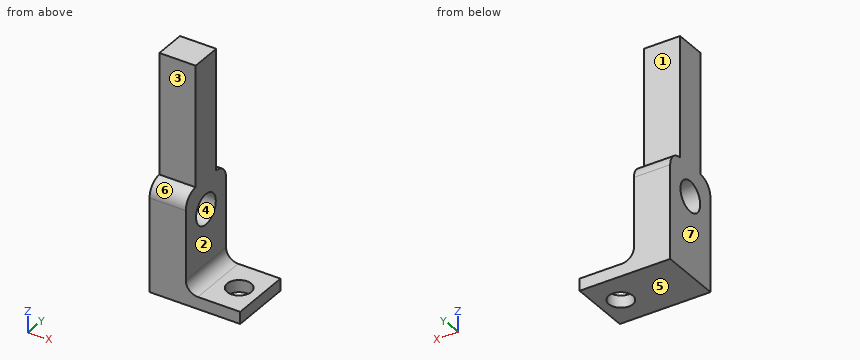
Autodesk Fusion 360 part; units mm, degrees
sketch "Sketch1" plane through (0, 0, 0) normal (0, 0, 1) x (1, 0, 0)
  line L0 (0, 0) -> (32, 0)
  line L1 (32, 0) -> (32, 10.2)
  line L2 (32, 10.2) -> (0, 10.2)
  line L3 (0, 10.2) -> (0, 0)
  dimension "d1" = 32
  dimension "d2" = 10.2
extrude "Extrude1" add sketch "Sketch1" along normal blind 2
sketch "Sketch2" plane through (0, 0, 2) normal (0, 0, 1) x (-1, 0, 0)
  line L0 (0, -10.2) -> (0, 0)
  line L1 (0, 0) -> (-32, 0)
  line L2 (-32, 0) -> (-32, -10.2)
  line L3 (-32, -10.2) -> (0, -10.2)
  line L4 (-7, -10.2) -> (-25, -10.2)
  line L5 (-25, -10.2) -> (-25, 0)
  line L6 (-25, 0) -> (-7, 0)
  line L7 (-7, 0) -> (-7, -10.2)
  circle A0 centre (-3.5, -5.1) radius 2
  circle A1 centre (-28.5, -5.1) radius 2
  dimension "d5" = 7
  dimension "d6" = 7
  dimension "d7" = 5.1
  dimension "d8" = 3.5
  dimension "d9" = 4
  dimension "d10" = 3.5
  dimension "d11" = 5.1
  dimension "d12" = 4
extrude "Extrude2" cut sketch "Sketch2" against normal blind 2.1 contours A0 | A1
extrude "Extrude3" add sketch "Sketch2" along normal blind 16 contours L1 L3 L4 L5 L6 L7
sketch "Sketch3" plane through (25, 0, 0) normal (1, 0, 0) x (0, 1, 0)
  line L0 (0, 2) -> (10.2, 2)
  line L1 (10.2, 2) -> (10.2, 18)
  line L2 (10.2, 18) -> (0, 18)
  line L3 (0, 18) -> (0, 2)
  circle A0 centre (5.1, 13) radius 2.5
  dimension "d17" = 5
  dimension "d18" = 5.1
  dimension "d19" = 5
extrude "Extrude4" cut sketch "Sketch3" against normal blind 20 contours A0
fillet "Fillet1" radius 2.5 2 edges at (16, 0, 18) (16, 10.2, 18)
fillet "Fillet2" radius 0.25 2 edges at (25, 5.1, 2) (7, 5.1, 2)
sketch "Sketch4" plane through (0, 0, 0) normal (0, -1, 0) x (1, 0, 0)
  line L0 (25, 15.5) -> (7, 15.5)
  line L1 (7, 15.5) -> (7, 2.25)
  arc A0 (6.75, 2) -> (7, 2.25) centre (6.75, 2.25) ccw
  line L2 (6.75, 2) -> (0, 2)
  line L3 (0, 2) -> (0, 0)
  line L4 (0, 0) -> (32, 0)
  line L5 (32, 0) -> (32, 2)
  line L6 (32, 2) -> (25.25, 2)
  arc A1 (25, 2.25) -> (25.25, 2) centre (25.25, 2.25) ccw
  line L7 (25, 2.25) -> (25, 15.5)
  line L8 (15.0115, 13.8918) -> (15.2499, 13.8388)
  line L9 (15.0115, 1.9217) -> (15.2499, 1.8688)
  line L10 (15.2499, 2.3085) -> (10.5625, 8.1981)
  line L11 (10.6841, 8.3354) -> (15.2499, 13.4918)
  line L12 (10.817, 8.3354) -> (15.3124, 13.4128)
  line L13 (15.3132, 2.3954) -> (10.6954, 8.1981)
  spline S0 degree 5 poles (15.0115, 13.8918) (15.0366, 13.8331) (15.0755, 13.7537) (15.1214, 13.6739) (15.1743, 13.5935) (15.2341, 13.5126) (15.2499, 13.4918) knots 0 0 0 0 0 0 0.04 0.053771 0.053771 0.053771 0.053771 0.053771 0.053771
  line L14 (15.2177, 13.5342) -> (15.2821, 13.4495)
  spline S1 degree 5 poles (15.2499, 2.3085) (15.2476, 2.3054) (15.194, 2.2294) (15.1434, 2.1527) (15.0959, 2.0753) (15.0514, 1.9972) (15.0115, 1.9217) knots 0.958261 0.958261 0.958261 0.958261 0.958261 0.958261 0.96 1 1 1 1 1 1
  line L15 (15.2777, 2.3478) -> (15.2221, 2.2693)
  line L16 (19.8903, 8.1981) -> (19.6849, 7.759)
  line L17 (19.6849, 7.759) -> (20.8035, 8.2887)
  line L18 (20.8035, 8.2887) -> (19.6849, 8.7197)
  line L19 (19.6849, 8.7197) -> (19.8674, 8.3354)
  spline S2 degree 5 poles (15.2499, 13.8388) (15.275, 13.7801) (15.3328, 13.6621) (15.4428, 13.4833) (15.636, 13.2415) (15.9534, 12.9319) (16.3409, 12.6103) (16.7857, 12.2676) (17.2659, 11.8886) (17.7534, 11.4561) (18.2174, 10.9546) (18.6276, 10.3741) (18.9469, 9.734) (19.126, 9.1768) (19.2132, 8.7476) (19.2502, 8.4653) (19.263, 8.3354) knots 0 0 0 0 0 0 0.04 0.08 0.12 0.16 0.2 0.24 0.28 0.32 0.36 0.4 0.44 0.473865 0.473865 0.473865 0.473865 0.473865 0.473865
  line L20 (19.1848, 9.1287) -> (19.3411, 7.542)
  spline S3 degree 5 poles (19.2746, 8.1981) (19.2853, 8.0482) (19.2958, 7.7438) (19.2774, 7.2862) (19.1846, 6.69) (18.9625, 5.9984) (18.6463, 5.3801) (18.2572, 4.8452) (17.8198, 4.3863) (17.3603, 3.9873) (16.904, 3.6275) (16.4734, 3.2862) (16.0845, 2.9471) (15.7463, 2.6009) (15.5197, 2.3146) (15.375, 2.094) (15.2897, 1.9443) (15.2499, 1.8688) knots 0.481014 0.481014 0.481014 0.481014 0.481014 0.481014 0.52 0.56 0.6 0.64 0.68 0.72 0.76 0.8 0.84 0.88 0.92 0.96 1 1 1 1 1 1
  line L21 (19.2097, 9.1087) -> (19.3396, 7.2875)
  spline S4 degree 5 poles (15.3124, 13.4128) (15.332, 13.3889) (15.4036, 13.3041) (15.5393, 13.1573) (15.762, 12.9459) (16.1025, 12.6633) (16.5474, 12.3206) (17.0276, 11.9416) (17.515, 11.5091) (17.979, 11.0075) (18.3892, 10.427) (18.7131, 9.7778) (18.894, 9.2098) (18.9811, 8.7693) (19.0172, 8.476) (19.0296, 8.3354) knots 0.064218 0.064218 0.064218 0.064218 0.064218 0.064218 0.08 0.12 0.16 0.2 0.24 0.28 0.32 0.36 0.4 0.44 0.476625 0.476625 0.476625 0.476625 0.476625 0.476625
  line L22 (14.9219, 13.8881) -> (15.7028, 12.9376)
  line L23 (18.9651, 9.0672) -> (19.094, 7.6035)
  spline S5 degree 5 poles (19.0398, 8.1981) (19.0483, 8.0587) (19.0561, 7.765) (19.0358, 7.3185) (18.9432, 6.7334) (18.7242, 6.0513) (18.408, 5.433) (18.0189, 4.8982) (17.5814, 4.4393) (17.1219, 4.0403) (16.6657, 3.6805) (16.235, 3.3392) (15.8681, 3.0192) (15.6141, 2.7622) (15.4485, 2.5703) (15.3521, 2.4471) (15.3132, 2.3954) knots 0.483768 0.483768 0.483768 0.483768 0.483768 0.483768 0.52 0.56 0.6 0.64 0.68 0.72 0.76 0.8 0.84 0.88 0.92 0.948678 0.948678 0.948678 0.948678 0.948678 0.948678
  line L24 (18.989, 9.0312) -> (19.0905, 7.3649)
  line L25 (15.7537, 2.9821) -> (14.8727, 1.8087)
  line L26 (10.6954, 8.1981) -> (19.0398, 8.1981)
  line L27 (19.2746, 8.1981) -> (19.8903, 8.1981)
  line L28 (19.263, 8.3354) -> (19.8674, 8.3354)
  line L29 (10.6725, 8.3354) -> (10.3002, 8.665)
  line L30 (10.3002, 8.665) -> (9.1473, 8.665)
  line L31 (9.1473, 8.665) -> (9.409, 8.2777)
  line L32 (9.409, 8.2777) -> (9.1615, 7.917)
  line L33 (9.1615, 7.917) -> (10.3, 7.917)
  line L34 (10.3, 7.917) -> (10.5625, 8.1981)
  line L35 (10.6725, 8.3354) -> (10.6841, 8.3354)
  line L36 (10.817, 8.3354) -> (19.0296, 8.3354)
  point P0 (16.3357, 12.6206)
  point P1 (16.627, 3.4048)
  point P2 (18.7456, 10.1048)
  point P3 (18.825, 5.7617)
  point P4 (18.5867, 5.8147)
  point P5 (18.5072, 10.1578)
  point P6 (16.0973, 12.6736)
  point P7 (16.3886, 3.4577)
extrude "Extrude5" cut sketch "Sketch4" against normal blind 0.3 contours L8 L9 S0 L14 S1 L15 S2 L20 S3 L21 S4 L22 L23 S5 L24 L25 | L16 L17 L18 L19 L20 L21 L27 L28 | L10 L11 L12 L13 L14 L15 L22 L23 L24 L25 L26 L29 L30 L31 L32 L33 L34 L35 L36
sketch "Sketch5" plane through (0, 0, 0) normal (0, -1, 0) x (1, 0, 0)
  line L0 (7, 15.5) -> (23, 15.5)
  line L1 (23, 15.5) -> (23, 0)
  line L2 (23, 0) -> (7, 0)
  line L3 (7, 0) -> (7, 15.5)
  line L4 (32, 0) -> (0, 0)
  point P0 (7, 15.5)
extrude "Extrude6" add sketch "Sketch4" sketch "Sketch5" against normal blind 1 contours L0 L1 A0 L2 L3 L4 L5 L6 A1 L7 | L8 L9 S0 L14 S1 L15 S2 L20 S3 L21 S4 L22 L23 S5 L24 L25 | L16 L17 L18 L19 L20 L21 L27 L28 | L10 L11 L12 L13 L14 L15 L22 L23 L24 L25 L26 L29 L30 L31 L32 L33 L34 L35 L36 | L13 S5 L26 of sketch 2
sketch "Sketch6" plane through (0, 0, 0) normal (0, -1, 0) x (1, 0, 0)
  line L0 (25, 15.5) -> (7, 15.5)
  line L1 (7, 15.5) -> (7, 2.25)
  arc A0 (6.75, 2) -> (7, 2.25) centre (6.75, 2.25) ccw
  line L2 (6.75, 2) -> (0, 2)
  line L3 (0, 2) -> (0, 0)
  line L4 (0, 0) -> (32, 0)
  line L5 (32, 0) -> (32, 2)
  line L6 (32, 2) -> (25.25, 2)
  arc A1 (25, 2.25) -> (25.25, 2) centre (25.25, 2.25) ccw
  line L7 (25, 2.25) -> (25, 15.5)
  line L8 (0, 20) -> (17, 20)
  line L9 (17, 20) -> (17, 0)
  line L10 (17, 0) -> (0, 0)
  line L11 (0, 0) -> (0, 20)
  dimension "d32" = 17
extrude "Extrude7" cut sketch "Sketch6" against normal blind 12 contours L0 L1 A0 L2 L3 L4 L9 L10 L11 | L0 L1 A0 L2 L8 L9 L11
sketch "Sketch7" plane through (0, 0, 0) normal (0, -1, 0) x (1, 0, 0)
  line L0 (17, 15.5) -> (17, 0)
  line L1 (17, 0) -> (32, 0)
  line L2 (32, 0) -> (32, 2)
  line L3 (32, 2) -> (25.25, 2)
  arc A0 (25, 2.25) -> (25.25, 2) centre (25.25, 2.25) ccw
  line L4 (25, 2.25) -> (25, 15.5)
  line L5 (25, 15.5) -> (17, 15.5)
  line L6 (23, 18) -> (25.1716, 18)
  line L7 (25.1716, 18) -> (25.1716, 2)
  line L8 (25.1716, 2) -> (23, 2)
  line L9 (23, 2) -> (23, 18)
  line L10 (25, 18) -> (17, 18)
  dimension "d35" = 2
extrude "Extrude8" cut sketch "Sketch7" against normal blind 12 contours A0 L4 L5 L6 L7 L9 L10 | A0 L4 L5 L7 L8 L9
sketch "Sketch8" plane through (0, 10.2, 0) normal (0, 1, 0) x (-1, 0, 0)
  line L0 (-23, 15.5) -> (-23, 2)
  line L1 (-23, 2) -> (-25.1716, 2)
  line L2 (-25.1716, 2) -> (-25.1716, 2.0126)
  arc A0 (-25.25, 2) -> (-25.1716, 2.0126) centre (-25.25, 2.25) ccw
  line L3 (-25.25, 2) -> (-32, 2)
  line L4 (-32, 2) -> (-32, 0)
  line L5 (-32, 0) -> (-17, 0)
  line L6 (-17, 0) -> (-17, 15.5)
  line L7 (-17, 15.5) -> (-23, 15.5)
  line L8 (-25.2855, 2) -> (-25.1, 2)
  line L9 (-25.1, 2) -> (-25.1, 2.05)
  line L10 (-25.1, 2.05) -> (-25.2855, 2.05)
  line L11 (-25.2855, 2.05) -> (-25.2855, 2)
extrude "Extrude9" cut sketch "Sketch8" against normal blind 12 contours L1 L2 A0 L3 L8 L9 L10 L11 | L2 A0 L8
fillet "Fillet3" radius 2 1 edges at (23, 5.1, 2)
extrude "Extrude10" add 1 faces at (21, 4.2333, 18) along direction (0, 0, 1) blind 20
Build history of the part. All positions in model axes, mm. Face numbers are marked on the shaded views. A direction names the side the tool comes from. Round coordinates to 2 decimals unless told otherwise and drop trailing zeros. Loops run counter-clockwise (first coordinate to the right, second up) from the corner with the lowest first, then second, coordinate; pieces in that order, holes last.
Item 1: Drill centre lines: line 1 along X through (y, z) = (5.1, 0.65); line 2 along Y through (x, z) = (28.5, 1.5); line 3 along Z through (x, y) = (18.5, 5.25). Where is each one in solid material? Low to high.
Item 2: Two-plate mould, pull along Z, no slides. Class the marked faces 4, 5, 6 and 7: released by +Z, released by -Z, zero draft, split by the parting line, or undercut.
Item 3: Saw through at C-C (z = 13). List the corners of the cut face in (x, y), then the cut area to 3 significant figures.
Item 4: Pin check, flat tips, straight feed: P1, Ø6.5, axis at x = 21, z = 28, coming from the -Y side; P2, Ø6, axis at y = 8.5, z = 21.5, coming from the +X side; P3, Ø3.5, axis at x = 29, y = 6, coming from the +Z side. Stop position of each tip, or through.
Item 5: Saw through at A-A (x = 28.5). List the corners of the cut face in (y, z), then the cut area to 3 significant figures.
Item 6: Which spindle directions (+Z, -Z, +X, -X, +Y, -Y) get a long thin tool onto all of the face, cutting with end or side? Do the marked faces 1, 2 and 3. Say none if no direction does.
Item 7: Saw through at B-B (y = 5.1). List the corners of the cut face in (x, z).
Item 8: Saw through at D-D (x = 18.5). List the corners of the cut face in (y, z).
Worked answers:
1. line 1: x = 17 to 26.5, 30.5 to 32
1. line 2: y = 0 to 3.1, 7.1 to 10.2
1. line 3: z = 0 to 10.5, 15.5 to 38
2. face 4: undercut
2. face 5: released by -Z
2. face 6: released by +Z
2. face 7: zero draft
3. outline: (17, 0) - (23, 0) - (23, 2.6) - (17, 2.6) - close; (17, 7.6) - (23, 7.6) - (23, 10.2) - (17, 10.2) - close
3. area: 31.2 mm2
4. P1: stops at y = 2.5
4. P2: stops at x = 23
4. P3: stops at z = 2
5. outline: (0, 0) - (3.1, 0) - (3.1, 2) - (0, 2) - close; (7.1, 0) - (10.2, 0) - (10.2, 2) - (7.1, 2) - close
5. area: 12.4 mm2
6. face 1: +Z, +X, -X, +Y
6. face 2: +Z, +X, +Y, -Y
6. face 3: +Z, +X, -X, -Y
7. outline: (17, 0) - (26.5, 0) - (26.5, 2) - (25, 2) arc R2 cw to (23, 4) - (23, 10.5) - (17, 10.5) - close; (17, 15.5) - (23, 15.5) - (23, 38) - (17, 38) - close; (30.5, 0) - (32, 0) - (32, 2) - (30.5, 2) - close
8. outline: (0, 0) - (10.2, 0) - (10.2, 15.5) arc R2.5 ccw to (7.7, 18) - (7.7, 38) - (2.5, 38) - (2.5, 18) arc R2.5 ccw to (0, 15.5) - close; hole circle Ø5 at (5.1, 13)
